For this review, take the finished solid that the model builds, in its own axes (mm). Face numbers are marked on the shaded views. A direction names the side the tool comes from. Give positions to 0.01 mm unless a question says otherwise; leave off trailing zeros. Loops run counter-clockwise (first coordinate to the right, second up) from the corner with the lowest first, then second, coordinate; pieces in that order, holes last. Notation, with made-up numbers: (66.25, -3.5) - (77.25, -3.5) arc R23 ccw to (77.25, 4.5) - close; hole circle Ø3 at (57.25, 53.5). An arc over 180 degrees is marked (long way). Put each result on its own line as item: value.
from build123d import *

# Parameters (mm, degrees)
SKETCH1_R           = 2.5
BOSS_EXTRUDE1_DEPTH = 5
SKETCH2_W           = 71.44
SKETCH2_H           = 5
BOSS_EXTRUDE2_DEPTH = 35


with BuildPart() as part:
    # Sketch1 → Boss-Extrude1 (new body)
    with BuildSketch(Plane.XY):
        with BuildLine():
            Line((-92.029607558, 58.476854566), (-105, 0))
            Line((-105, 0), (0, 0))
            Line((0, 0), (0, 75))
            Line((0, 75), (-71.44, 75))
            ThreePointArc((-71.44, 75), (-84.639870022, 70.358450729), (-92.029607558, 58.476854566))
        make_face()
        with Locations((-71.44, 53.91)):
            Circle(SKETCH1_R, mode=Mode.SUBTRACT)
    extrude(amount=BOSS_EXTRUDE1_DEPTH)

    # Sketch2 → Boss-Extrude2 (add)
    with BuildSketch(Plane.XY.offset(5)):
        Polygon((-105, 0), (-92.029607558, 58.476854566), (-87.14824019, 57.39414841), (-99.878484221, 0), align=None)
        with Locations((-35.72, 72.5)):
            Rectangle(SKETCH2_W, SKETCH2_H)
    extrude(amount=-BOSS_EXTRUDE2_DEPTH)


solid = part.part
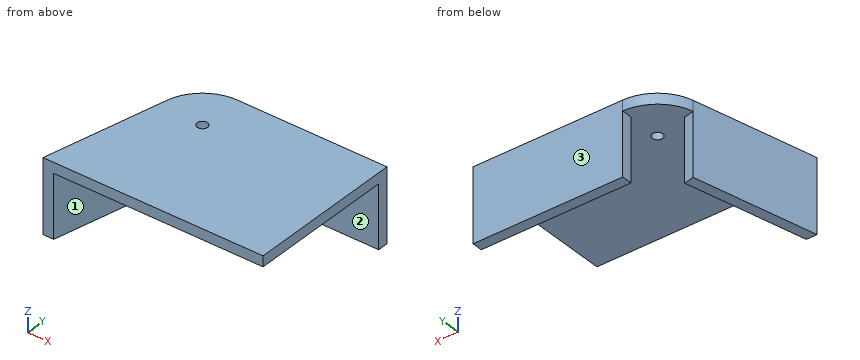
1) Take a section at D-D on y = 35. State the section outline as (x, z) points, and give its area (3 significant figures).
Geometry check:
outline: (-97.24, -30) - (-92.12, -30) - (-92.12, 0) - (0, 0) - (0, 5) - (-97.24, 5) - close
area: 640 mm²
2) Wall thickness on line 1 (Y direction, x = -55, z = -13.5); line 2 (Z direction, x = -33.5, y = 43); line 3 (X direction, y = 53, z = 2): over which ranges is each line inside the solid? List them lowest first.
Geometry check:
line 1: y = 70 to 75
line 2: z = 0 to 5
line 3: x = -93.24 to -73.77, -69.11 to 0
3) Take a section at A-A on z = -14.5. State the section outline as (x, y) points, and give its area (3 significant figures).
Geometry check:
outline: (-105, 0) - (-99.88, 0) - (-87.15, 57.39) - (-92.03, 58.48) - close; (-71.44, 70) - (0, 70) - (0, 75) - (-71.44, 75) - close
area: 654 mm²
4) Take a section at B-B on y = 53.91. State the section outline as (x, z) points, and give its area (3 significant figures).
Geometry check:
outline: (-93.04, -30) - (-87.92, -30) - (-87.92, 0) - (-73.94, 0) - (-73.94, 5) - (-93.04, 5) - close; (-68.94, 0) - (0, 0) - (0, 5) - (-68.94, 5) - close
area: 594 mm²
5) For the marked faces 1, 2 and 3, list the 3-axis set-ups (+Z, -Z, +X, -X, +Y, -Y) from which the entire face can be reached by the end or side of a thin tool; tool diameter is ignored.
Geometry check:
face 1: -Z, +X, -Y
face 2: -Z, +X, -X, -Y
face 3: +Z, -Z, +X, -X, +Y
6) Insertion check: pin 1 Ø2 at (x, z) = (-89.5, -9) entering from +Y; pin 2 Ø4 at (y, z) = (54, -22) entering from +X; pin 3 Ø5.5 at (y, z) = (72.5, -21.5) entering from -X; pin 4 Ø3 at (x, y) = (-71.44, 53.91) entering from -Z. Each pin has a flat end and moves straight along its axis. Give the tip position at first contact, or say it passes through.
Geometry check:
pin 1: stops at y = 58.14
pin 2: stops at x = -87.46
pin 3: stops at x = -71.44
pin 4: passes through
7) Take a section at C-C on x = -41. State the section outline as (y, z) points.
Geometry check:
outline: (0, 0) - (70, 0) - (70, -30) - (75, -30) - (75, 5) - (0, 5) - close
